Design review of the part built by this model. Coordinates are the model's own, in mm. Coordinates: 2 decimals unless noted, no trailing zeros. Loops run counter-clockwise (first coordinate to the right, second up) from the corner with the lowest first, then second, coordinate; pieces in that order, holes last. Notation, with made-up numbers: (84, 85) -> (91, 85) arc R14 cw to (91, 104) -> close; hole circle Ø8 at (78.25, 25.25). An arc over 180 degrees is marked (long way). Answer in a Markdown table with one row per item.
```python
from build123d import *

# Parameters (mm, degrees)
BOSS_EXTRUDE1_DEPTH     = 5
FILLET1_R               = 7.5
CUT_EXTRUDE2_DEPTH      = 183.030179489
CUT_EXTRUDE2_DEPTH_BACK = 183.030179489
SKETCH3_R               = 1.6
CUT_EXTRUDE3_DEPTH      = 183.030179489
CUT_EXTRUDE3_DEPTH_BACK = 183.030179489
SKETCH4_R               = 25
SKETCH4_R_2             = 1.6
CUT_EXTRUDE4_DEPTH      = 183.030179489
CUT_EXTRUDE4_DEPTH_BACK = 183.030179489
SKETCH5_R               = 1.6
CUT_EXTRUDE5_DEPTH      = 183.030179489
CUT_EXTRUDE5_DEPTH_BACK = 183.030179489
SKETCH6_R               = 1.6


with BuildPart() as part:
    # Sketch1 → Boss-Extrude1 (new body)
    with BuildSketch(Plane(origin=(0, 0, 0), x_dir=(1, 0, 0), z_dir=(0, 1, 0))):
        with BuildLine():
            Line((115, 67.5), (133.954283246, 67.5))
            ThreePointArc((133.954283246, 67.5), (106.066017178, 106.066017178), (67.5, 133.954283246))
            Line((67.5, 133.954283246), (67.5, 115))
            Line((67.5, 115), (-67.5, 115))
            Line((-67.5, 115), (-67.5, 133.954283246))
            ThreePointArc((-67.5, 133.954283246), (-106.066017178, 106.066017178), (-133.954283246, 67.5))
            Line((-133.954283246, 67.5), (-115, 67.5))
            Line((-115, 67.5), (-115, -67.5))
            Line((-115, -67.5), (-133.954283246, -67.5))
            ThreePointArc((-133.954283246, -67.5), (-106.066017178, -106.066017178), (-67.5, -133.954283246))
            Line((-67.5, -133.954283246), (-67.5, -115))
            Line((-67.5, -115), (67.5, -115))
            Line((67.5, -115), (67.5, -133.954283246))
            ThreePointArc((67.5, -133.954283246), (106.066017178, -106.066017178), (133.954283246, -67.5))
            Line((133.954283246, -67.5), (115, -67.5))
            Line((115, -67.5), (115, 67.5))
        make_face()
    extrude(amount=BOSS_EXTRUDE1_DEPTH)

    # Fillet1
    fillet1_edges = [part.edges().sort_by_distance(p)[0] for p in [
        (-67.5, 2.5, 133.954283246),
        (-133.954283246, 2.5, 67.5),
        (-133.954283246, 2.5, -67.5),
        (-67.5, 2.5, -133.954283246),
        (67.5, 2.5, -133.954283246),
        (133.954283246, 2.5, -67.5),
        (133.954283246, 2.5, 67.5),
        (67.5, 2.5, 133.954283246),
    ]]
    fillet(fillet1_edges, radius=FILLET1_R)

    # Sketch3 → Cut-Extrude2 (cut, two sides: drawn at the far end of the back side and taken through both)
    with BuildSketch(Plane(origin=(0, 5, 0), x_dir=(1, 0, 0), z_dir=(0, 1, 0)).offset(-CUT_EXTRUDE2_DEPTH_BACK)):
        with Locations(Location((-15, -95, 0), (0, 0, 270))):
            Circle(SKETCH3_R)
        with Locations(Location((-15, -65, 0), (0, 0, 270))):
            Circle(SKETCH3_R)
        with Locations(Location((15, -65, 0), (0, 0, 270))):
            Circle(SKETCH3_R)
        with Locations(Location((15, -95, 0), (0, 0, 270))):
            Circle(SKETCH3_R)
        with Locations(Location((-65, 15, 0), (0, 0, 270))):
            Circle(SKETCH3_R)
        with Locations(Location((-65, -15, 0), (0, 0, 270))):
            Circle(SKETCH3_R)
        with Locations(Location((-95, -15, 0), (0, 0, 270))):
            Circle(SKETCH3_R)
        with Locations(Location((-95, 15, 0), (0, 0, 270))):
            Circle(SKETCH3_R)
        with Locations(Location((15, 65, 0), (0, 0, 270))):
            Circle(SKETCH3_R)
        with Locations(Location((-15, 65, 0), (0, 0, 270))):
            Circle(SKETCH3_R)
        with Locations(Location((-15, 95, 0), (0, 0, 270))):
            Circle(SKETCH3_R)
        with Locations(Location((15, 95, 0), (0, 0, 270))):
            Circle(SKETCH3_R)
        with Locations(Location((65, -15, 0), (0, 0, 270))):
            Circle(SKETCH3_R)
        with Locations(Location((65, 15, 0), (0, 0, 270))):
            Circle(SKETCH3_R)
        with Locations(Location((95, 15, 0), (0, 0, 270))):
            Circle(SKETCH3_R)
        with Locations(Location((95, -15, 0), (0, 0, 270))):
            Circle(SKETCH3_R)
    extrude(amount=CUT_EXTRUDE2_DEPTH + CUT_EXTRUDE2_DEPTH_BACK, mode=Mode.SUBTRACT)

    # Sketch4 → Cut-Extrude3 (cut, two sides: drawn at the far end of the back side and taken through both)
    with BuildSketch(Plane(origin=(0, 5, 0), x_dir=(1, 0, 0), z_dir=(0, 1, 0)).offset(-CUT_EXTRUDE3_DEPTH_BACK)):
        with Locations(Location((0, 0, 0), (0, 0, 270))):
            Circle(SKETCH4_R)
        with Locations(Location((0, 30, 0), (0, 0, 270))):
            Circle(SKETCH4_R_2)
        with Locations(Location((21.213203436, 21.213203436, 0), (0, 0, 270))):
            Circle(SKETCH4_R_2)
        with Locations(Location((30, 0, 0), (0, 0, 270))):
            Circle(SKETCH4_R_2)
        with Locations(Location((21.213203436, -21.213203436, 0), (0, 0, 270))):
            Circle(SKETCH4_R_2)
        with Locations(Location((0, -30, 0), (0, 0, 270))):
            Circle(SKETCH4_R_2)
        with Locations(Location((-21.213203436, -21.213203436, 0), (0, 0, 270))):
            Circle(SKETCH4_R_2)
        with Locations(Location((-30, 0, 0), (0, 0, 270))):
            Circle(SKETCH4_R_2)
        with Locations(Location((-21.213203436, 21.213203436, 0), (0, 0, 270))):
            Circle(SKETCH4_R_2)
    extrude(amount=CUT_EXTRUDE3_DEPTH + CUT_EXTRUDE3_DEPTH_BACK, mode=Mode.SUBTRACT)

    # Sketch5 → Cut-Extrude4 (cut, two sides: drawn at the far end of the back side and taken through both)
    with BuildSketch(Plane(origin=(0, 5, 0), x_dir=(1, 0, 0), z_dir=(0, 1, 0)).offset(-CUT_EXTRUDE4_DEPTH_BACK)):
        with Locations(Location((75, -75, 0), (0, 0, 270))):
            Circle(SKETCH5_R)
        with Locations(Location((-75, -75, 0), (0, 0, 270))):
            Circle(SKETCH5_R)
        with Locations(Location((75, 75, 0), (0, 0, 270))):
            Circle(SKETCH5_R)
        with Locations(Location((-75, 75, 0), (0, 0, 270))):
            Circle(SKETCH5_R)
    extrude(amount=CUT_EXTRUDE4_DEPTH + CUT_EXTRUDE4_DEPTH_BACK, mode=Mode.SUBTRACT)

    # Sketch6 → Cut-Extrude5 (cut, two sides: drawn at the far end of the back side and taken through both)
    with BuildSketch(Plane(origin=(0, 5, 0), x_dir=(1, 0, 0), z_dir=(0, 1, 0)).offset(-CUT_EXTRUDE5_DEPTH_BACK)):
        with Locations(Location((-113.890872965, -85.606601718, 0), (0, 0, 270))):
            Circle(SKETCH6_R)
        with Locations(Location((-85.606601718, -113.890872965, 0), (0, 0, 270))):
            Circle(SKETCH6_R)
        with Locations(Location((-113.890872965, 85.606601718, 0), (0, 0, 270))):
            Circle(SKETCH6_R)
        with Locations(Location((-85.606601718, 113.890872965, 0), (0, 0, 270))):
            Circle(SKETCH6_R)
        with Locations(Location((85.606601718, 113.890872965, 0), (0, 0, 270))):
            Circle(SKETCH6_R)
        with Locations(Location((113.890872965, 85.606601718, 0), (0, 0, 270))):
            Circle(SKETCH6_R)
        with Locations(Location((113.890872965, -85.606601718, 0), (0, 0, 270))):
            Circle(SKETCH6_R)
        with Locations(Location((85.606601718, -113.890872965, 0), (0, 0, 270))):
            Circle(SKETCH6_R)
    extrude(amount=CUT_EXTRUDE5_DEPTH + CUT_EXTRUDE5_DEPTH_BACK, mode=Mode.SUBTRACT)


solid = part.part
```
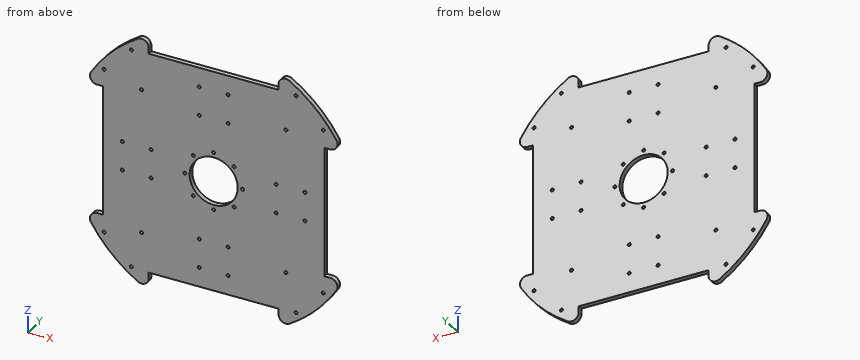
(1) To check wall thickness, follow probe 1 along X at (y, z) = (2.4, 0); probe 2 along X at (y, z) = (2.45, -75); probe 3 along Z at (x, y) = (-65, 3.6). State the ranges of each line that lie inside material, in increasing order.
Evaluation:
| item | result |
|---|---|
| probe 1 | x = -115 to -31.6, -28.4 to -25, 25 to 28.4, 31.6 to 115 |
| probe 2 | x = -128.67 to -76.6, -73.4 to 73.4, 76.6 to 128.67 |
| probe 3 | z = -115 to -16.6, -13.4 to 13.4, 16.6 to 115 |
(2) Take a section at B-B on x = -108. Give the boundary of the cut face in (y, z), and give its area (3 significant figures).
Evaluation:
| item | result |
|---|---|
| outline | (0, -104.1) -> (5, -104.1) -> (5, 104.1) -> (0, 104.1) -> close |
| area | 1,040 mm² |
(3) For pin 1 (1.5 mm diameter, centred on y = 2, z = -90, fed in from -X); pin 2 (1.5 mm diameter, centred on x = 118.5, y = 3, fed in from +Z); pin 3 (3 mm diameter, centred on y = 1.5, z = -53, fed in from -X), all flat-tipped, find the tip position at first contact; note any pin that passes through.
Evaluation:
| item | result |
|---|---|
| pin 1 | stops at x = -120.56 |
| pin 2 | stops at z = 92.92 |
| pin 3 | stops at x = -115 |
(4) Take a section at A-A on y = 3.45. Count the separate pieces of the cut face and the enclosed holes in it, and give its area (3 significant figures).
Evaluation:
| item | result |
|---|---|
| separate pieces | 1 |
| enclosed holes | 37 |
| area | 52,000 mm² |
